Autodesk Inventor part; units mm, degrees
ref_plane "YZ Plane" through (0, 0, 0) normal (1, 0, 0) x (0, 1, 0)
ref_plane "XZ Plane" through (0, 0, 0) normal (0, 1, 0) x (-1, 0, 0)
ref_plane "XY Plane" through (0, 0, 0) normal (0, 0, 1) x (1, 0, 0)
sketch "Sketch1" plane through (0, 0, 0) normal (1, 0, 0) x (0, 1, 0)
  circle A0 centre (0, 0) radius 7.9375
  arc A1 (-3.3867, 25.1732) -> (3.3867, -25.1732) centre (0, 0) ccw
  line L0 (3.3867, -25.1732) -> (192.1857, 0.2268)
  line L1 (0, -25.4) -> (385.0288, -25.4) construction
  circle A2 centre (56.6397, 7.62) radius 31.75 construction
  line L2 (56.6397, 7.62) -> (47.1998, 6.35) construction
  line L3 (57.9097, -1.82) -> (48.4698, -3.09)
  line L4 (45.9298, 15.79) -> (55.3697, 17.06)
  arc A3 (57.9097, -1.82) -> (55.3697, 17.06) centre (56.6397, 7.62) ccw
  arc A4 (45.9298, 15.79) -> (48.4698, -3.09) centre (47.1998, 6.35) ccw
  circle A5 centre (188.7991, 25.4) radius 50.8 construction
  circle A6 centre (188.7991, 25.4) radius 14.2875
  line L5 (137.4291, -7.1399) -> (134.7624, 12.6815) construction
  line L6 (134.7624, 12.6815) -> (95.1195, 7.3482) construction
  line L7 (95.1195, 7.3482) -> (97.7862, -12.4732) construction
  circle A7 centre (47.1998, 6.35) radius 31.75 construction
  line L8 (76.8346, -7.7854) -> (67.3947, -9.0554) construction
  line L9 (76.4926, -5.2429) -> (67.0526, -6.5129)
  line L10 (67.7367, -11.5979) -> (77.1767, -10.3279)
  arc A8 (77.1767, -10.3279) -> (76.4926, -5.2429) centre (76.8346, -7.7854) ccw
  arc A9 (67.0526, -6.5129) -> (67.7367, -11.5979) centre (67.3947, -9.0554) ccw
  line L11 (36.4448, 23.0254) -> (27.0049, 21.7554) construction
  line L12 (36.1028, 25.5679) -> (26.6628, 24.2979)
  line L13 (27.3469, 19.2129) -> (36.7869, 20.4829)
  arc A10 (36.7869, 20.4829) -> (36.1028, 25.5679) centre (36.4448, 23.0254) ccw
  arc A11 (26.6628, 24.2979) -> (27.3469, 19.2129) centre (27.0049, 21.7554) ccw
  line L14 (56.6397, 7.62) -> (76.8346, -7.7854) construction
  line L15 (56.6397, 7.62) -> (36.4448, 23.0254) construction
  line L16 (56.6397, 7.62) -> (88.1062, 11.8533) construction
  circle A12 centre (126.185, 1.4375) radius 2.5527
  circle A13 centre (106.3636, -1.2292) radius 2.5527
  line L17 (126.185, 1.4375) -> (106.3636, -1.2292) construction
  line L18 (126.185, 1.4375) -> (136.0957, 2.7708) construction
  line L19 (106.3636, -1.2292) -> (96.4529, -2.5625) construction
  line L20 (0, 0) -> (239.1455, 32.1733) construction
  arc A14 (192.1857, 0.2268) -> (185.4124, 50.5732) centre (188.7991, 25.4) ccw
  line L21 (185.4124, 50.5732) -> (-3.3867, 25.1732)
  point P0 (51.9197, 6.985)
  point P1 (72.1146, -8.4204)
  point P2 (31.7249, 22.3904)
  dimension "d1" = 63.5
  dimension "d5" = 101.6
  dimension "d0" = 15.875
  dimension "d2" = 50.8
  dimension "d3" = 9.525
  dimension "d4" = 9.525
  dimension "d6" = 28.575
  dimension "d8" = 20
  dimension "d9" = 40
  dimension "d11" = 2.5654
  dimension "d12" = 25.4
  dimension "d15" = 25.4
  dimension "d16" = 45
  dimension "d17" = 47.625
  dimension "d18" = 6.35
  dimension "d19" = 5.1054
  dimension "d20" = 20
  dimension "d21" = 241.3
extrude "Extrusion1" add sketch "Sketch1" along normal blind 6.35
properties part number "Arm Plates"
Build history of the part. All positions in model axes, mm. Give positions to 0.01 mm unless a question says otherwise; leave off trailing zeros. Loops run counter-clockwise (first coordinate to the right, second up) from the corner with the lowest first, then second, coordinate; pieces in that order, holes last. Notation, with made-up numbers: (89.5, 83) -> (102.5, 83) arc R18 ccw to (102.5, 107) -> close; hole circle Ø3 at (85.5, -18). An arc over 180 degrees is marked (long way). One line per question, with ' | ' between items. Start each with the question number.
1) Two-plate mould, pull along Y, no slides. Class faces 1 (the flat face through (3.13, 92.33, 38.05)), 2 (the flat face through (3.131, 50.584, 16.416)), 3 (the flat face through (3.13, 96.46, -12.65)): released by +Y, released by -Y, zero draft, split by the parting line, or undercut.
2) Cut at A-A (y = 0). Give the cut face in (x, z), plus the area to 3 significant figures.
3) Cut at B-B (x = 5.25). Count the separate pieces of the cut face and the enclosed holes in it, plus the area to 3 significant figures.
4) Cut at C-C (z = 31.5). Give the cut face in (x, y), plus the area to 3 significant figures.
5) Pin check, flat tips, straight feed: pin 1 (3 mm diameter, centred on x = 1, z = 14, fed in from -Y); pin 2 (5 mm diameter, centred on y = 166.5, z = -7, fed in from +X); pin 3 (1 mm diameter, centred on x = 4.5, z = 41, fed in from +Y); pin 4 (2 mm diameter, centred on x = 2, z = -5.5, fed in from -Y). Stop position of each tip, or through.
6) Probe L1, parallel to Z at x = 3.5, y = 0; L2, parallel to Z at x = 2.25, y = 61; L3, parallel to Y at x = 2.5, z = 11. List the from-to ranges inside material, lowest first.
Return value:
1) face 1: released by -Y | face 2: undercut | face 3: released by +Y
2) outline: (0, -25.4) -> (6.35, -25.4) -> (6.35, -7.94) -> (0, -7.94) -> close; (0, 7.94) -> (6.35, 7.94) -> (6.35, 25.63) -> (0, 25.63) -> close | area: 223 mm^2
3) separate pieces: 1 | enclosed holes: 7 | area: 10,200 mm^2
4) outline: (0, 43.64) -> (6.35, 43.64) -> (6.35, 175.88) -> (0, 175.88) -> close; (0, 201.72) -> (6.35, 201.72) -> (6.35, 213.46) -> (0, 213.46) -> close | area: 914 mm^2
5) pin 1: y = -22.11 | pin 2: through | pin 3: y = 209.22 | pin 4: y = -25
6) L1: -25.4 to -7.94, 7.94 to 25.63 | L2: -17.42 to -0.85, 16.09 to 33.84 | L3: -22.89 to 38.89, 65.54 to 209.72
